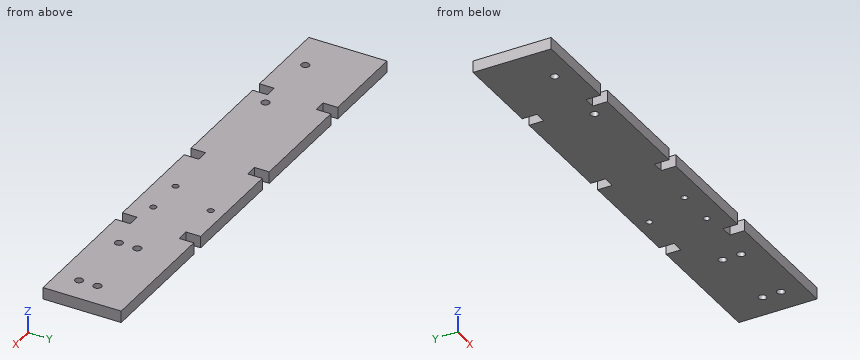
from build123d import *

# Parameters (mm, degrees)
F0_W     = 240
F0_H     = 40
F1_DEPTH = 6
F2_W     = 6.2
F2_H     = 7.5
F3_DEPTH = 6
F4_R     = 1.6
F5_R     = 2.05
F6_R     = 2.05
F7_DEPTH = 6.001
F8_DEPTH = 6.001


with BuildPart() as f1:
    # F0 (on Top) → F1 (new body)
    with BuildSketch(Plane.XY):
        with Locations((10.5305, 0)):
            Rectangle(F0_W, F0_H)
    extrude(amount=F1_DEPTH)

    # F2 (on face) → F3 (cut, through all)
    with BuildSketch(Plane.XY.offset(6)):
        with Locations((0, -16.25)):
            Rectangle(F2_W, F2_H)
        with Locations((-61.9, -16.25)):
            Rectangle(F2_W, F2_H)
        with Locations((61.9, -16.25)):
            Rectangle(F2_W, F2_H)
        with Locations((0, 16.25)):
            Rectangle(F2_W, F2_H)
        with Locations((-61.9, 16.25)):
            Rectangle(F2_W, F2_H)
        with Locations((61.9, 16.25)):
            Rectangle(F2_W, F2_H)
    extrude(amount=-F3_DEPTH, mode=Mode.SUBTRACT)

    # F4 (on face) + F5 (on face) + F6 (on face) → F7 (cut, through all)
    with BuildSketch(Plane.XY.offset(6)):
        with Locations((27.860826, -10.4)):
            Circle(F4_R)
        with Locations((47.860826, -10.4)):
            Circle(F4_R)
        with Locations((37.860826, 13.3)):
            Circle(F4_R)
    with BuildSketch(Plane.XY.offset(6)):
        with Locations((-88.650754, -10)):
            Circle(F5_R)
        with Locations((-52.650754, -10)):
            Circle(F5_R)
    with BuildSketch(Plane.XY.offset(6)):
        with Locations((81.389095, -9)):
            Circle(F6_R)
        with Locations((117.389095, -9)):
            Circle(F6_R)
        with Locations((81.389095, 0.4)):
            Circle(F6_R)
        with Locations((117.389095, 0.4)):
            Circle(F6_R)
    extrude(amount=-F7_DEPTH, mode=Mode.SUBTRACT)

    # F6 (on face) + F5 (on face) + F4 (on face) → F8 (cut, through all)
    with BuildSketch(Plane.XY.offset(6)):
        with Locations((81.389095, -9)):
            Circle(F6_R)
        with Locations((117.389095, -9)):
            Circle(F6_R)
        with Locations((81.389095, 0.4)):
            Circle(F6_R)
        with Locations((117.389095, 0.4)):
            Circle(F6_R)
    with BuildSketch(Plane.XY.offset(6)):
        with Locations((-88.650754, -10)):
            Circle(F5_R)
        with Locations((-52.650754, -10)):
            Circle(F5_R)
    with BuildSketch(Plane.XY.offset(6)):
        with Locations((27.860826, -10.4)):
            Circle(F4_R)
        with Locations((47.860826, -10.4)):
            Circle(F4_R)
        with Locations((37.860826, 13.3)):
            Circle(F4_R)
    extrude(amount=-F8_DEPTH, mode=Mode.SUBTRACT)


solid = f1.part
Input: part model. Units: mm. Frame: model coordinates. Round coordinates to 2 decimals unless told otherwise and drop trailing zeros. Order: outer loops, then holes, each group sorted by start corner. A loop starts at its lowest first (then second) coordinate and runs counter-clockwise, first axis right, second up. Notation, with made-up numbers: (-8, 40) - (15, 40) arc R26 ccw to (15, 60) - close; hole circle Ø7 at (7, 20.25). An arc over 180 degrees is marked (long way). Use a Markdown table: item, result.
1. Section B-B on z = 4. State how many separate pieces and enclosed holes the cut face has, then the cut area to 3 significant figures.
Evaluation:
| item | result |
|---|---|
| separate pieces | 1 |
| enclosed holes | 9 |
| area | 9,220 mm^2 |
2. Material intervals for probe 1 along X at (y, z) = (15.5, 0.7); probe 2 along Y at (x, z) = (-53, 1.6); probe 3 along Y at (x, z) = (115.5, 5.75), sorted ascending.
Evaluation:
| item | result |
|---|---|
| probe 1 | -109.47 to -65, -58.8 to -3.1, 3.1 to 58.8, 65 to 130.53 |
| probe 2 | -20 to -12.02, -7.98 to 20 |
| probe 3 | -20 to -9.8, -8.2 to -0.4, 1.2 to 20 |
3. Section A-A on y = 0.4. Return the cut outline in (x, z), then the cut area to 3 significant figures.
Evaluation:
| item | result |
|---|---|
| outline | (-109.47, 0) - (79.34, 0) - (79.34, 6) - (-109.47, 6) - close; (83.44, 0) - (115.34, 0) - (115.34, 6) - (83.44, 6) - close; (119.44, 0) - (130.53, 0) - (130.53, 6) - (119.44, 6) - close |
| area | 1,390 mm^2 |
